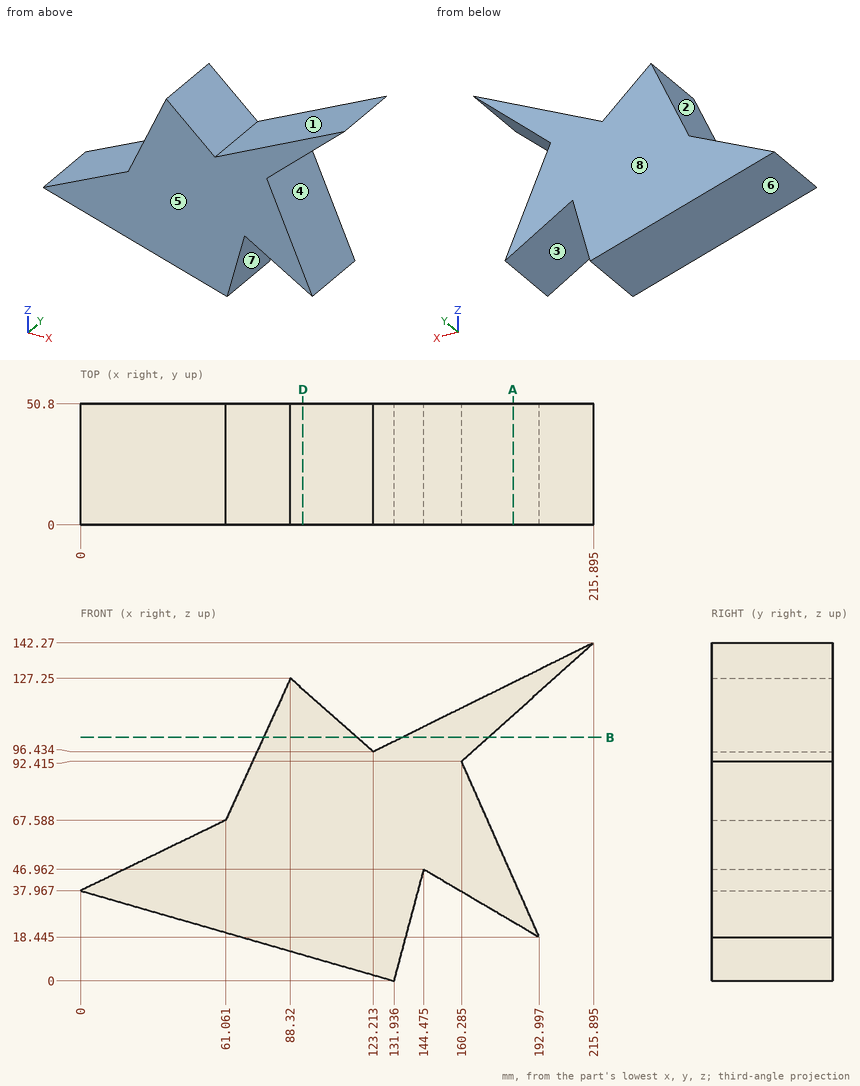
Part print with two shaded views. Sizes in mm from the minimum x, y, z corner. A direction names the side the tool comes from. Round coordinates to 2 decimals unless told otherwise and drop trailing zeros. Order: outer loops, then holes, each group sorted by start corner. A loop starts at its lowest first (then second) coordinate and runs counter-clockwise, first axis right, second up. Notation, with made-up numbers: (1, 39) - (10, 39) arc R14 cw to (10, 61) - close; hole circle Ø1 at (88.5, 53). An arc over 180 degrees is marked (long way). Answer in a Markdown table with one row per item. Add a question column.
(1) Band-saw the part on A-A on x = 182. List the corners of the cut face in (y, z), and give its area (3 significant figures).
(2) Probe L1, parallel to X at y = 16, z = 127 (1 decimal); L2, parallel to Z at x = 173, y = 9.5 (1 decimal); L3, parallel to Z at x = 186.5, y = 22.5 (1 decimal). List the from-to ranges inside material, lowest first. Write a range as [from, to].
(3) Band-saw the part on B-B on z = 102.5. List the corners of the cut face in (x, y).
(4) 3-axis set-ups, long thin cutter, end or side, ignore diameter. For the marked faces 1, 2, 3, 4 and 5: which of +Z, -Z, +X, -X, +Y, -Y reach the whole face in a straight line?
(5) Drop flat-ended pins along their axis: pin 1 Ø1 at (x, y) = (79, 29.5) entering from -Z; pin 2 Ø3 at (x, y) = (23.5, 20) entering from +Z (1 decimal); pin 3 Ø5 at (x, y) = (94, 12.5) entering from -Z. Give the stop position or say it passes through.
(6) Mould opens along X. For the marked faces 6, 7 and 8 say: +X half, -X half, draft (parallel to the pull), parting line (faces both ways), or undercut.
(7) Band-saw the part on D-D on x = 93.5. List the corners of the cut face in (y, z) (1 decimal).
Data:
| question | item | result |
|---|---|---|
| 1 | outline | (0, 24.91) - (50.8, 24.91) - (50.8, 43.31) - (0, 43.31) - close; (0, 111.88) - (50.8, 111.88) - (50.8, 125.51) - (0, 125.51) - close |
| 1 | area | 1,630 mm^2 |
| 2 | L1 | x = [88.2, 88.6], [185, 198.9] |
| 2 | L2 | z = [30.2, 63.7], [103.8, 121.1] |
| 2 | L3 | z = [22.3, 33.1], [115.9, 127.7] |
| 3 | outline | (77.01, 0) - (116.34, 0) - (116.34, 50.8) - (77.01, 50.8) - close; (135.48, 0) - (171.53, 0) - (171.53, 50.8) - (135.48, 50.8) - close |
| 4 | face 1 | +Z, +Y, -Y |
| 4 | face 2 | +Z, -X, +Y, -Y |
| 4 | face 3 | -Z, +Y, -Y |
| 4 | face 4 | +X, +Y, -Y |
| 4 | face 5 | +Z, -Z, +X, -X, -Y |
| 5 | pin 1 | stops at z = 15.09 |
| 5 | pin 2 | stops at z = 50.1 |
| 5 | pin 3 | stops at z = 10.2 |
| 6 | face 6 | -X half |
| 6 | face 7 | undercut |
| 6 | face 8 | draft |
| 7 | outline | (0, 11.1) - (50.8, 11.1) - (50.8, 122.7) - (0, 122.7) - close |
